from build123d import *

# Parameters (mm, degrees)
F0_W     = 254
F0_H     = 203.2
F1_DEPTH = 19.05
F2_R     = 38.1
F2_W     = 558.8
F2_H     = 19.05
F3_DEPTH = 228.6
F4_W     = 254
F4_H     = 203.2
F4_W_2   = 57.15
F5_DEPTH = 19.05


with BuildPart() as f1:
    # F0 (on Front) → F1 (new body)
    with BuildSketch(Plane.XZ):
        with BuildLine():
            Line((0, -203.2), (0, 0))
            Line((0, 0), (-431.8, 0))
            ThreePointArc((-431.8, 0), (-491.3159020629, -143.6840979371), (-635, -203.2))
            Line((-635, -203.2), (0, -203.2))
        make_face()
        with BuildLine():
            Line((-635, -203.2), (-635, 0))
            Line((-635, 0), (-838.2, 0))
            ThreePointArc((-838.2, 0), (-778.6840979371, -143.6840979371), (-635, -203.2))
        make_face()
        with BuildLine():
            ThreePointArc((-635, -203.2), (-491.3159020629, -143.6840979371), (-431.8, 0))
            Line((-431.8, 0), (-635, 0))
            Line((-635, 0), (-635, -203.2))
        make_face()
        with Locations((127, -101.6)):
            Rectangle(F0_W, F0_H)
    extrude(amount=F1_DEPTH)

    # F2 (on face) → F3 (join)
    with BuildSketch(Plane.XZ.offset(19.05)):
        with Locations((152.4, -101.6)):
            Circle(F2_R)
        Polygon((-57.15, -203.2), (-57.15, 0), (-76.2, 0), (-76.2, -184.15), (-76.2, -203.2), align=None)
        with Locations((-355.6, -193.675)):
            Rectangle(F2_W, F2_H)
        with BuildLine():
            Line((-635, -203.2), (-635, -184.15))
            ThreePointArc((-635, -184.15), (-765.2137137555, -130.2137137555), (-819.15, 0))
            Line((-819.15, 0), (-838.2, 0))
            ThreePointArc((-838.2, 0), (-778.6840979371, -143.6840979371), (-635, -203.2))
        make_face()
    extrude(amount=F3_DEPTH)

    # F4 (on face) → F5 (join)
    with BuildSketch(Plane.XZ.offset(247.65)):
        with Locations((127, -101.6)):
            Rectangle(F4_W, F4_H)
        with Locations((-28.575, -101.6)):
            Rectangle(F4_W_2, F4_H)
        with BuildLine():
            ThreePointArc((-838.2, 0), (-778.6840979371, -143.6840979371), (-635, -203.2))
            Line((-635, -203.2), (-635, -184.15))
            ThreePointArc((-635, -184.15), (-765.2137137555, -130.2137137555), (-819.15, 0))
            Line((-819.15, 0), (-838.2, 0))
        make_face()
        with BuildLine():
            Line((-635, -184.15), (-635, 0))
            Line((-635, 0), (-819.15, 0))
            ThreePointArc((-819.15, 0), (-765.2137137555, -130.2137137555), (-635, -184.15))
        make_face()
        with BuildLine():
            Line((-76.2, -184.15), (-76.2, 0))
            Line((-76.2, 0), (-431.8, 0))
            ThreePointArc((-431.8, 0), (-463.6153953484, -109.1675651849), (-549.0987922087, -184.15))
            Line((-549.0987922087, -184.15), (-76.2, -184.15))
        make_face()
        with BuildLine():
            Line((-57.15, -203.2), (-57.15, 0))
            Line((-57.15, 0), (-76.2, 0))
            Line((-76.2, 0), (-76.2, -184.15))
            Line((-76.2, -184.15), (-549.0987922087, -184.15))
            ThreePointArc((-549.0987922087, -184.15), (-591.0059094877, -198.380341768), (-635, -203.2))
            Line((-635, -203.2), (-57.15, -203.2))
        make_face()
        with BuildLine():
            Line((-635, -184.15), (-635, -203.2))
            ThreePointArc((-635, -203.2), (-591.0059094877, -198.380341768), (-549.0987922087, -184.15))
            Line((-549.0987922087, -184.15), (-635, -184.15))
        make_face()
        with BuildLine():
            ThreePointArc((-549.0987922087, -184.15), (-463.6153953484, -109.1675651849), (-431.8, 0))
            Line((-431.8, 0), (-635, 0))
            Line((-635, 0), (-635, -184.15))
            Line((-635, -184.15), (-549.0987922087, -184.15))
        make_face()
    extrude(amount=F5_DEPTH)


solid = f1.part
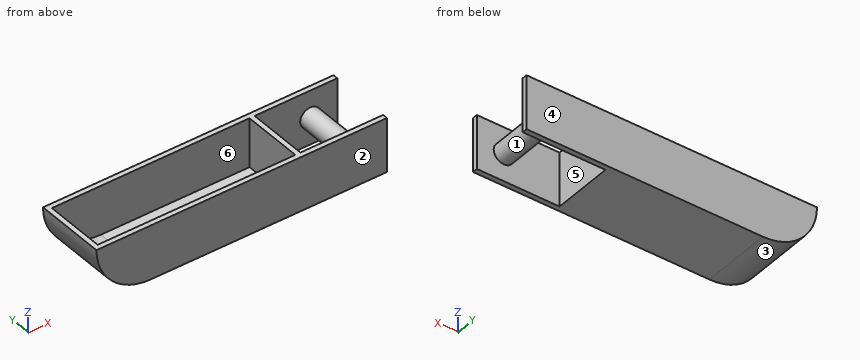
Verification items for the finished model (mm, model axes). Face numbers are marked on the shaded views. A direction names the side the tool comes from. Give positions to 0.01 mm unless a question says otherwise; leave off trailing zeros. Write each loop counter-clockwise with the first axis right and the second up, starting at its lowest first coordinate (ties: lowest second). Pieces come first, ordered by that corner, then holes. Notation, with made-up numbers: M 1.5,89.25 L 60.5,89.25 A32 cw 60.5,125.25 Z; hole C 85,-25 d4. An arc over 180 degrees is marked long. Write item = value, one per line.
(1) Material ranges on line 1 (Y direction, x = 167, z = -38.5); line 2 (X direction, y = -208, z = -116); line 3 (X direction, y = -82, z = -95.5), recorded low to high.
Found:
line_1 = -266.7 to -247.65, -19.05 to 0
line_2 = -801.84 to -778.02, -76.2 to -57.15, 117.13 to 187.67
line_3 = -814.36 to -792.45, -76.2 to -57.15, 114.79 to 190.01
(2) Sectioned sample at C-C (z = -15). Record the cut outline in (x, y).
Found:
outline = M -837.65,-266.7 L 254,-266.7 L 254,-247.65 L -57.15,-247.65 L -57.15,-19.05 L 254,-19.05 L 254,0 L -837.65,0 Z; hole M -818.54,-247.65 L -76.2,-247.65 L -76.2,-19.05 L -818.54,-19.05 Z
(3) Sectioned sample at A-A (x = 55.5). Record the cut outline in (y, z), then the cut area to 3 significant figures.
Found:
outline = M -266.7,-203.2 L -247.65,-203.2 L -247.65,0 L -266.7,0 Z; M -19.05,-203.2 L 0,-203.2 L 0,0 L -19.05,0 Z
area = 7,740 mm2
(4) Sectioned sample at B-B (y = -68). Record the cut outline in (x, z).
Found:
outline = M -838.2,0 A203.2 ccw -635,-203.2 L -57.15,-203.2 L -57.15,0 L -76.2,0 L -76.2,-184.15 L -635,-184.15 A184.15 cw -819.15,0 Z; C 152.4,-101.6 d76.2
(5) Sectioned sample at D-D (x = -646). Record the cut outline in (y, z).
Found:
outline = M -266.7,-202.9 L 0,-202.9 L 0,0 L -19.05,0 L -19.05,-183.82 L -247.65,-183.82 L -247.65,0 L -266.7,0 Z
(6) Draft check along Y on the marked faces 1, 2 and 3. Enter one of: released by +Y, released by -Y, zero draft, split by the parting line, or undercut.
Found:
face_1 = undercut
face_2 = released by -Y
face_3 = zero draft
(7) Access from +Z, -Z, +X, -X, +Y, -Y to the whole of each face (thin tool, end or side, straight path). Record for the marked faces 4, 5 and 6.
Found:
face_4 = +Z, -Z, +X, -X, +Y
face_5 = +Z, -Z
face_6 = +Z
(8) Go/stop test with flat-tipped pins: pin 1 Ø1 at (y, z) = (-114.5, -25.5) entering from -X; pin 2 Ø8 at (y, z) = (-143.5, -55) entering from -X; pin 3 Ø2 at (x, y) = (-661, -155) entering from +Z. Record where each tip stops, or that it passes through.
Found:
pin_1 = -836.66
pin_2 = -831.7
pin_3 = -182.16
